Geometry check sheet. Reference: the model listing, model coordinates, mm. Round coordinates to 2 decimals unless told otherwise and drop trailing zeros. Order: outer loops, then holes, each group sorted by start corner. A loop starts at its lowest first (then second) coordinate and runs counter-clockwise, first axis right, second up. Notation, with made-up numbers: (-22, -39) - (24, -39) arc R16 cw to (24, -22) - close; hole circle Ø7 at (8, 32). An arc over 180 degrees is marked (long way). Use a Markdown table: item, result. Add a question column.
(1) Mould release check, pull along X, two halves, no side actions. Record for faces 1 (the face through (38.552, 10.664, 0.246)), 2 (the face through (-2.579, -1.978, 0.246)), 3 (the face through (-1, 10, 0)): released by +X, released by -X, zero draft, split by the parting line, or undercut.
(2) Section check A-A on z = 0.2. Record the boundary of the cut face in (x, y) (3 decimals), then the cut area to 3 significant figures.
(3) Gauge pin test, flat end, axial feed: P1, Ø2.5, axis at x = 14.25, y = 0, coming from the -Z side. Record the tip position at first contact, or that the pin passes through.
(4) Section check C-C on y = -13. Record the boundary of the cut face in (x, z).
(5) Section check B-B on x = 0. Record the boundary of the cut face in (y, z), then the cut area to 3 significant figures.
(6) Section check D-D on y = 0. Record the boundary of the cut face in (x, z).
(7) Thickness scan on line 1 along X through (y, z) = (0, 0.35); line 2 along Y through (x, z) = (0, 0.3); line 3 along X through (y, z) = (-27, 0.1). Record the ranges inside material, lowest first. Write a range as [from, to].
```python
from build123d import *

# Parameters (mm, degrees)
SKETCH001_R     = 40
PAD_DEPTH       = 0.5
SKETCH_W        = 32.5
SKETCH_H        = 12
POCKET_DEPTH    = 0.501
SKETCH002_R     = 3.25
SKETCH002_R_2   = 1.5
POCKET001_DEPTH = 0.501
SKETCH003_R     = 1
POCKET002_DEPTH = 0.501
SKETCH004_W     = 3
SKETCH004_H     = 3.42
SKETCH004_H_2   = 2.91
PAD001_DEPTH    = 0.5
SKETCH005_R     = 4.42
PAD002_DEPTH    = 0.5


with BuildPart() as part:
    # Sketch001 → Pad (new body)
    with BuildSketch(Plane.XY):
        Circle(SKETCH001_R)
    extrude(amount=PAD_DEPTH)

    # Sketch → Pocket (cut, through all)
    with BuildSketch(Plane.XY):
        with Locations((0, -23)):
            Rectangle(SKETCH_W, SKETCH_H)
    extrude(amount=POCKET_DEPTH, mode=Mode.SUBTRACT)

    # Sketch002 → Pocket001 (cut, through all)
    with BuildSketch(Plane.XY):
        Circle(SKETCH002_R)
        with Locations((14.25, 0)):
            Circle(SKETCH002_R_2)
        with Locations((-14.25, 0)):
            Circle(SKETCH002_R_2)
    extrude(amount=POCKET001_DEPTH, mode=Mode.SUBTRACT)

    # Sketch003 → Pocket002 (cut, through all)
    with BuildSketch(Plane.XY):
        with Locations((-26, -13)):
            Circle(SKETCH003_R)
    extrude(amount=POCKET002_DEPTH, mode=Mode.SUBTRACT)

    # Sketch004 → Pad001 (join)
    with BuildSketch(Plane.XY):
        with Locations((0, -40.81)):
            Rectangle(SKETCH004_W, SKETCH004_H)
        with Locations((0, 40.675)):
            Rectangle(SKETCH004_W, SKETCH004_H_2)
    extrude(amount=PAD001_DEPTH)

    # Sketch005 → Pad002 (join)
    with BuildSketch(Plane.XY):
        with Locations((18.565, -32.63)):
            Circle(SKETCH005_R)
        with Locations((-18.565, -32.63)):
            Circle(SKETCH005_R)
    extrude(amount=PAD002_DEPTH)


solid = part.part
```
Check sheet entries:
| question | item | result |
|---|---|---|
| 1 | face 1 | released by +X |
| 1 | face 2 | undercut |
| 1 | face 3 | zero draft |
| 2 | outline | (-22.984, -32.738) arc R4.42 ccw to (-16.4, -36.483) arc R40 ccw to (-1.5, -39.972) - (-1.5, -42.52) - (1.5, -42.52) - (1.5, -39.972) arc R40 ccw to (16.4, -36.483) arc R4.42 ccw to (22.984, -32.738) arc R40 ccw to (1.5, 39.972) - (1.5, 42.13) - (-1.5, 42.13) - (-1.5, 39.972) arc R40 ccw to start; hole circle Ø2 at (-26, -13); hole (-16.25, -28.865) arc R4.42 cw to (-16.043, -29) - (16.043, -29) arc R4.42 cw to (16.25, -28.865) - (16.25, -17) - (-16.25, -17) - close; hole circle Ø3 at (-14.25, 0); hole circle Ø6.5 at (0, 0); hole circle Ø3 at (14.25, 0) |
| 2 | area | 4,620 mm2 |
| 3 | P1 | passes through |
| 4 | outline | (-37.83, 0) - (-27, 0) - (-27, 0.5) - (-37.83, 0.5) - close; (-25, 0) - (37.83, 0) - (37.83, 0.5) - (-25, 0.5) - close |
| 5 | outline | (-42.52, 0) - (-29, 0) - (-29, 0.5) - (-42.52, 0.5) - close; (-17, 0) - (-3.25, 0) - (-3.25, 0.5) - (-17, 0.5) - close; (3.25, 0) - (42.13, 0) - (42.13, 0.5) - (3.25, 0.5) - close |
| 5 | area | 33.1 mm2 |
| 6 | outline | (-40, 0) - (-15.75, 0) - (-15.75, 0.5) - (-40, 0.5) - close; (-12.75, 0) - (-3.25, 0) - (-3.25, 0.5) - (-12.75, 0.5) - close; (3.25, 0) - (12.75, 0) - (12.75, 0.5) - (3.25, 0.5) - close; (15.75, 0) - (40, 0) - (40, 0.5) - (15.75, 0.5) - close |
| 7 | line 1 | x = [-40, -15.75], [-12.75, -3.25], [3.25, 12.75], [15.75, 40] |
| 7 | line 2 | y = [-42.52, -29], [-17, -3.25], [3.25, 42.13] |
| 7 | line 3 | x = [-29.51, -16.25], [16.25, 29.51] |
